Design review of the part built by this model. Coordinates are the model's own, in mm. Face numbers are marked on the shaded views. A direction names the side the tool comes from. Give positions to 0.01 mm unless a question says otherwise; leave off trailing zeros. Order: outer loops, then holes, each group sorted by start corner. A loop starts at its lowest first (then second) coordinate and runs counter-clockwise, first axis right, second up. Notation, with made-up numbers: M 60.25,66 L 108.25,66 A31 ccw 108.25,97 Z; hole C -20.5,17.25 d4. An arc over 180 degrees is marked long. Put each result on its own line as item: value. Start each with the question number.
from build123d import *

# Parameters (mm, degrees)
SKETCH1_R                  = 34
MAINHOUSING_DEPTH          = 90
SKETCH2_R                  = 15
REARPART_DEPTH             = 10
SKETCH3_R                  = 6
SHAFT_DEPTH                = 9.5
SKETCH4_R                  = 10
GEAR_DEPTH                 = 3
HEXBOLT_DEPTH              = 8.7
SKETCH6_R                  = 10
SKETCH6_R_2                = 6
HEXBOLTCUTOUT_DEPTH        = 3.2
TOP_BOTTOMSEPERATION_START = 9
SKETCH7_R                  = 34
SKETCH7_R_2                = 33.9
TOP_BOTTOMSEPERATION_DEPTH = 72
SKETCH8_R                  = 2.5
SCREWHOLE_DEPTH            = 12.4
SCREWHOLEPATTERN_COUNT     = 3


with BuildPart() as part:
    # Sketch1 → MainHousing (new body)
    with BuildSketch(Plane(origin=(0, 0, 0), x_dir=(1, 0, 0), z_dir=(0, 1, 0))):
        Circle(SKETCH1_R)
    extrude(amount=MAINHOUSING_DEPTH)

    # Sketch2 → RearPart (add)
    with BuildSketch(Plane.XZ):
        Circle(SKETCH2_R)
    extrude(amount=REARPART_DEPTH)

    # Sketch3 → Shaft (add)
    with BuildSketch(Plane(origin=(0, 90, 0), x_dir=(1, 0, 0), z_dir=(0, 1, 0))):
        Circle(SKETCH3_R)
    extrude(amount=SHAFT_DEPTH)

    # Sketch4 → Gear (add)
    with BuildSketch(Plane(origin=(0, 99.5, 0), x_dir=(1, 0, 0), z_dir=(0, 1, 0))):
        Circle(SKETCH4_R)
    extrude(amount=GEAR_DEPTH)

    # Sketch5 → HexBolt (add)
    with BuildSketch(Plane(origin=(0, 102.5, 0), x_dir=(1, 0, 0), z_dir=(0, 1, 0))):
        Polygon((0, 6.92820323), (-6, 3.464101615), (-6, -3.464101615), (0, -6.92820323), (6, -3.464101615), (6, 3.464101615), align=None)
    extrude(amount=HEXBOLT_DEPTH)

    # Sketch6 → HexBoltCutout (cut)
    with BuildSketch(Plane(origin=(0, 102.5, 0), x_dir=(1, 0, 0), z_dir=(0, 1, 0))):
        Circle(SKETCH6_R)
        Circle(SKETCH6_R_2, mode=Mode.SUBTRACT)
    extrude(amount=HEXBOLTCUTOUT_DEPTH, mode=Mode.SUBTRACT)

    # Sketch7 → Top/BottomSeperation (cut)
    with BuildSketch(Plane(origin=(0, 0, 0), x_dir=(1, 0, 0), z_dir=(0, 1, 0)).offset(TOP_BOTTOMSEPERATION_START)):
        Circle(SKETCH7_R)
        Circle(SKETCH7_R_2, mode=Mode.SUBTRACT)
    extrude(amount=TOP_BOTTOMSEPERATION_DEPTH, mode=Mode.SUBTRACT)

    # Sketch8 → ScrewHole (cut)
    with BuildSketch(Plane(origin=(0, 90, 0), x_dir=(1, 0, 0), z_dir=(0, 1, 0))):
        with Locations((0, 22)):
            Circle(SKETCH8_R)
    screwhole = extrude(amount=-SCREWHOLE_DEPTH, mode=Mode.SUBTRACT)

    # ScrewHolePattern: ScrewHole ×3 about axis
    screwholepattern_axis = Axis((0, 0, 0), (0, 1, 0))
    for i in range(1, SCREWHOLEPATTERN_COUNT):
        add(screwhole.rotate(screwholepattern_axis, i * 360 / SCREWHOLEPATTERN_COUNT), mode=Mode.SUBTRACT)


solid = part.part
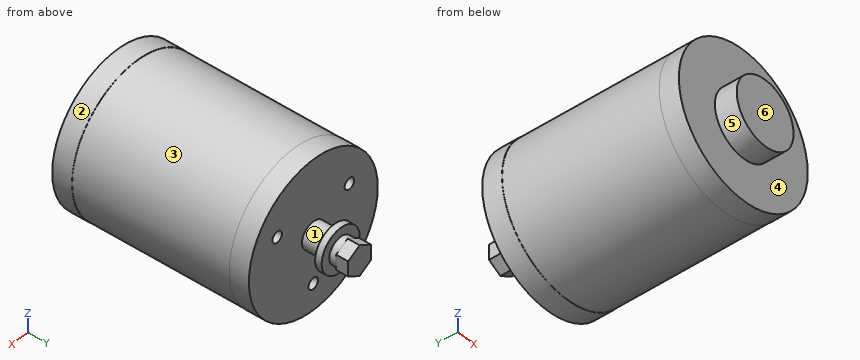
1. The part is to be moulded in two halves that separate along Y. For the marked faces 1, 2, 3 and 4, say which applies: +Y half, -Y half, draft (parallel to the pull), parting line (faces both ways), or undercut.
2. Consider section A-A on x = 26. Give the boundary of the cut face in (y, z).
3. Machinability: for the marked faces 5 and 6, which of the approach directions +Z, -Z, +X, -X, +Y, -Y give a long, thin tool a straight path to every point of the face, cutting with its end or side? Answer none if there is none.
4. Consider section D-D on y = 83.5. Give the boundary of the cut face in (x, z).
5. To check wall thickness, follow probe 1 along Y at (x, z) = (-5, 4); probe 2 along Z at (x, y) = (0, 87); probe 3 along Y at (x, z) = (-2, 31.5). State the ranges of each line that lie inside material, in increasing order.
6. Consider section B-B on z = 18.5. Give the boundary of the cut face in (x, y), then the cut area to 3 significant figures.
7. Insertion check: pin 1 (8 mm diameter, centred on x = 5, y = 14, fed in from +Z); pin 2 (12 mm diameter, centred on x = 24, y = 14.5, fed in from +Z); pin 3 (6 mm diameter, centred on x = 10.5, y = 24.5, fed in from +Z). Each pin has a flat end and moves straight along its axis. Give the tip position at first contact, or say it passes through.
8. Consider section C-C on y = 46.5. Give the boundary of the cut face in (x, z).
Returned:
1. face 1: undercut
1. face 2: draft
1. face 3: undercut
1. face 4: -Y half
2. outline: M 0,-21.91 L 9,-21.91 L 9,-21.75 L 81,-21.75 L 81,-21.91 L 90,-21.91 L 90,21.91 L 81,21.91 L 81,21.75 L 9,21.75 L 9,21.91 L 0,21.91 Z
3. face 5: -Y
3. face 6: +Z, -Z, +X, -X, -Y
4. outline: C 0,0 d68; hole C -19.05,11 d5; hole C 0,-22 d5; hole C 19.05,11 d5
5. probe 1: y = -10 to 90, 99.5 to 102.5, 105.7 to 111.2
5. probe 2: z = -34 to -24.5, -19.5 to 34
5. probe 3: y = 0 to 90
6. outline: M -28.53,0 L 28.53,0 L 28.53,9 L 28.41,9 L 28.41,81 L 28.53,81 L 28.53,90 L -28.53,90 L -28.53,81 L -28.41,81 L -28.41,9 L -28.53,9 Z
6. area: 5,120 mm2
7. pin 1: stops at z = 33.89
7. pin 2: stops at z = 28.73
7. pin 3: stops at z = 33.06
8. outline: C 0,0 d67.8
